from build123d import *

# Parameters (mm, degrees)
SKETCH_W        = 34
SKETCH_H        = 10
PAD_DEPTH       = 7
POCKET_DEPTH    = 0.4
FILLET_R        = 1
POCKET001_DEPTH = 86.211236
CHAMFER_SIZE    = 0.5
SKETCH005_R     = 1.35
POCKET002_DEPTH = 7
POCKET003_DEPTH = 14.001


with BuildPart() as part:
    # Sketch (on XY_Plane of Origin) → Pad (new body, symmetric)
    with BuildSketch(Plane.XY):
        Rectangle(SKETCH_W, SKETCH_H)
    extrude(amount=PAD_DEPTH, both=True)

    # Sketch002 (on XY_Plane of Origin) → Pocket (cut)
    with BuildSketch(Plane.XY):
        Polygon((4.751306, -6.5), (11, 3.5), (-10.225191, 3.5), (-15.998694, -6.5), align=None)
    extrude(amount=-POCKET_DEPTH, mode=Mode.SUBTRACT)

    # Fillet
    fillet_edges = [part.edges().sort_by_distance(p)[0] for p in [
        (17, 0, 7),
        (17, 0, -7),
        (-17, 0, -7),
        (-17, 0, 7),
    ]]
    fillet(fillet_edges, radius=FILLET_R)

    # Sketch003 (on Face1 of Fillet) → Pocket001 (cut, through all)
    with BuildSketch(Plane.XZ.offset(5)):
        with BuildLine():
            ThreePointArc((3, 5.6), (1.4, 4), (3, 2.4))
            Line((3, 2.4), (13, 2.4))
            ThreePointArc((13, 2.4), (14.6, 4), (13, 5.6))
            Line((3, 5.6), (13, 5.6))
        make_face()
    pocket001 = extrude(amount=-POCKET001_DEPTH, mode=Mode.SUBTRACT)

    # Mirrored: Pocket001 across XY
    add(pocket001.mirror(Plane.XY), mode=Mode.SUBTRACT)

    # Chamfer
    chamfer_edges = [part.edges().sort_by_distance(p)[0] for p in [
        (0, 5, -7),
    ]]
    chamfer(chamfer_edges, length=CHAMFER_SIZE)

    # Sketch005 (on Face13 of Chamfer) → Pocket002 (cut)
    with BuildSketch(Plane.YZ.offset(17)):
        with Locations((-1, 0)):
            Circle(SKETCH005_R)
    extrude(amount=-POCKET002_DEPTH, mode=Mode.SUBTRACT)

    # Sketch006 (on Face7 of Pocket002) → Pocket003 (cut, through all)
    with BuildSketch(Plane(origin=(0, 0, -7), x_dir=(1, 0, 0), z_dir=(0, 0, -1))):
        Polygon((-4, 7), (0, 3), (22.51627, 3), (22.51627, 7), align=None)
    extrude(amount=-POCKET003_DEPTH, mode=Mode.SUBTRACT)


solid = part.part
Source: CAD feature listing. Evaluate the final solid. Frame: model axes, mm. A direction names the side the tool comes from. Round coordinates to 2 decimals unless told otherwise and drop trailing zeros. Loops run counter-clockwise (first coordinate to the right, second up) from the corner with the lowest first, then second, coordinate; pieces in that order, holes last. Notation, with made-up numbers: (6.5, 34.25) -> (12.5, 34.25) arc R20 ccw to (12.5, 66.25) -> close; hole circle Ø6 at (3.25, -2). An arc over 180 degrees is marked (long way). Answer as a JSON object with one key per item and string values. Group by question number.
Q1. Ray query, line 1 (Z direction, x = 12.5, y = -1); line 2 (Z direction, x = 13, y = -2.75); line 3 (Z direction, x = 3.5, y = -2.25). Return the intervals inside material, ascending. Write a range as from..to.
Q2. Section query B-B (z = 4). Output: boundary loops of the cut face in (x, y), plus the area to 3 significant figures.
Q3. Section query C-C (y = -2). Output: boundary loops of the cut face in (x, z).
Q4. Contact query for flat-ended pins moving along their axis: P1, Ø1.4, axis at y = -1, z = 0.5, coming from the +X side; P2, Ø6, axis at x = 0, z = 3.5, coming from the -Y side. Output: stop coordinate, or through.
Q5. Mould query, pull axis Z, two halves, no side actions, for faces 6 (the cylindrical face through (1.4, 0.9, -4)), 7 (the flat face through (0, 5, 0)), 8 (the cylindrical face through (16.699, 0.803, -6.715)). Classes: pulls with the +Z half, pulls with the -Z half, needs draft (parallel to the pull), parting line crosses it, or undercut.
Q6. Section query A-A (x = 6). Output: boundary loops of the cut face in (y, z).
Q7. Access query for faces 1 (the flat face through (8, -3, 0)), 2 (the flat face through (-17, 0, 0)), 3 (the flat face through (8, 1, 2.4)), 4 (the cylindrical face through (16.699, 0.803, 6.715)), 5 (the cylindrical face through (13.55, -2.07, -0.82)). Directions: +Z, -Z, +X, -X, +Y, -Y. A direction counts if a zero-diameter tool reaches every point of the face in a straight line with its end or side. Return the directions, or none.
Q8. Section query D-D (z = 0.5). Output: boundary loops of the cut face in (x, y), plus the area to 3 significant figures.
Completed:
{
 "1": {"line 1": "-7..-5.6, -2.4..-1.35, 1.35..2.4, 5.6..7", "line 2": "-7..-5.6, -2.4..2.4, 5.6..7", "line 3": "-7..-5.6, -2.4..-0.4, 0..2.4, 5.6..7"},
 "2": {"outline": "(-17, -5) -> (-2, -5) -> (0, -3) -> (1.4, -3) -> (1.4, 5) -> (-16.5, 5) -> (-17, 4.5) -> close; (14.6, -3) -> (17, -3) -> (17, 4.5) -> (16.5, 5) -> (14.6, 5) -> close", "area": "198 mm²"},
 "3": {"outline": "(-17, -6) arc R1 ccw to (-16, -7) -> (16, -7) arc R1 ccw to (17, -6) -> (17, -0.91) -> (10, -0.91) -> (10, 0.91) -> (17, 0.91) -> (17, 6) arc R1 ccw to (16, 7) -> (-16, 7) arc R1 ccw to (-17, 6) -> close; hole (-13.4, -0.4) -> (7.56, -0.4) -> (7.56, 0) -> (-13.4, 0) -> close; hole (3, -5.6) -> (13, -5.6) arc R1.6 ccw to (13, -2.4) -> (3, -2.4) arc R1.6 ccw to start; hole (3, 2.4) -> (13, 2.4) arc R1.6 ccw to (13, 5.6) -> (3, 5.6) arc R1.6 ccw to start"},
 "4": {"P1": "x = 10", "P2": "y = -5"},
 "5": {"face 6": "undercut", "face 7": "needs draft", "face 8": "pulls with the -Z half"},
 "6": {"outline": "(-3, -7) -> (4.5, -7) -> (5, -6.5) -> (5, -5.6) -> (-3, -5.6) -> close; (-3, -2.4) -> (5, -2.4) -> (5, 2.4) -> (-3, 2.4) -> (-3, 0) -> (3.5, 0) -> (3.5, -0.4) -> (-3, -0.4) -> close; (-3, 5.6) -> (5, 5.6) -> (5, 6.5) -> (4.5, 7) -> (-3, 7) -> close"},
 "7": {"face 1": "+Z, -Z, +X, -Y", "face 2": "+Z, -Z, -X, +Y, -Y", "face 3": "+Y, -Y", "face 4": "+Z, +X, +Y, -Y", "face 5": "+X"},
 "8": {"outline": "(-17, -5) -> (-2, -5) -> (0, -3) -> (17, -3) -> (17, -2.25) -> (10, -2.25) -> (10, 0.25) -> (17, 0.25) -> (17, 4.5) -> (16.5, 5) -> (-16.5, 5) -> (-17, 4.5) -> close", "area": "286 mm²"}
}
